Build history of the part. All positions in model axes, mm. Face numbers are marked on the shaded views. A direction names the side the tool comes from. Round coordinates to 2 decimals unless told otherwise and drop trailing zeros. Write each loop counter-clockwise with the first axis right and the second up, starting at its lowest first coordinate (ties: lowest second). Pieces come first, ordered by that corner, then holes.
1) Saw through at C-C (x = -38.5). Write the cut outline in (y, z).
2) Saw through at A-A (x = -62.5). Write the cut outline in (y, z), plus the area to 3 significant figures.
3) Which spindle directions (+Z, -Z, +X, -X, +Y, -Y) get a long thin tool onto all of the face, cutting with end or side? Do the marked faces 5 and 6. Say none if no direction does.
4) Pull direction X, two halves, no side cores. Call the marked faces 1, 2, 3 and 4: +X half, -X half, draft (parallel to the pull), parting line (faces both ways), or undercut.
5) Flat gauge pins, fed straight in: pin 1 (1.5 mm diameter, centred on x = 10.5, z = 7, fed in from -Y); pin 2 (2.5 mm diameter, centred on x = 56, z = 4, fed in from +Y); pin 3 (3 mm diameter, centred on x = 8.5, z = 4, fed in from -Y). Where does each tip first touch, or does it go through?
6) Wall check: probe 1 along X at (y, z) = (3.25, 2); probe 2 along Y at (x, z) = (-55.5, 2.25); probe 3 along Y at (x, z) = (-51, 2.5). Give the ranges that are in metal, low to high.
7) Saw through at B-B (y = 7). Write the cut outline in (x, z), plus the area to 3 significant figures.
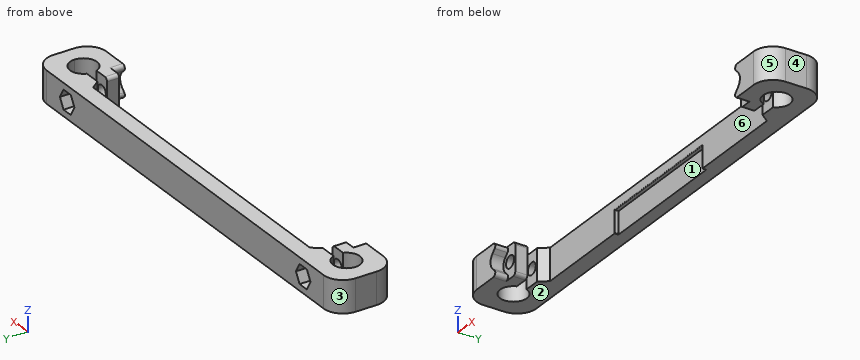
from build123d import *

# Parameters (mm, degrees)
SALIENTE_EXTRUIR1_DEPTH = 10
CROQUIS2_R              = 1.9
CORTAR_EXTRUIR1_DEPTH   = 25
CORTAR_EXTRUIR5_DEPTH   = 74.087139772
CROQUIS8_W              = 5.376990951
CROQUIS8_H              = 7.8
CORTAR_EXTRUIR6_DEPTH   = 74.087139772
CORTAR_EXTRUIR7_DEPTH   = 4.25
CROQUIS10_R             = 1.9
CORTAR_EXTRUIR8_DEPTH   = 4
REDONDEO1_R             = 1
CROQUIS11_W             = 41.47
CROQUIS11_H             = 14
CORTAR_EXTRUIR9_DEPTH   = 1.2
REDONDEO2_R             = 0.2


with BuildPart() as part:
    # Croquis1 → Saliente-Extruir1 (new body)
    with BuildSketch(Plane.XY):
        with BuildLine():
            Line((65.8, 9.3), (-65.8, 9.3))
            ThreePointArc((-65.8, 9.3), (-70.042640687, 7.542640687), (-71.8, 3.3))
            Line((-71.8, 3.3), (-71.8, -3.3))
            ThreePointArc((-71.8, -3.3), (-70.042640687, -7.542640687), (-65.8, -9.3))
            Line((-65.8, -9.3), (-48.2, -9.3))
            Line((-48.2, -9.3), (-48.2, -1.5))
            Line((-48.2, -1.5), (-58.576990951, -1.5))
            ThreePointArc((-58.576990951, -1.5), (-66.7, 0), (-58.576990951, 1.5))
            Line((-58.576990951, 1.5), (-46.2, 1.5))
            Line((-46.2, 1.5), (-46.2, -9.3))
            Line((-46.2, -9.3), (46.2, -9.3))
            Line((46.2, -9.3), (46.2, 1.5))
            Line((46.2, 1.5), (58.576990951, 1.5))
            ThreePointArc((58.576990951, 1.5), (63.26268014, 4.130171789), (66.7, 0))
            ThreePointArc((66.7, 0), (63.26268014, -4.130171789), (58.576990951, -1.5))
            Line((58.576990951, -1.5), (48.2, -1.5))
            Line((48.2, -1.5), (48.2, -9.3))
            Line((48.2, -9.3), (65.8, -9.3))
            ThreePointArc((65.8, -9.3), (70.042640687, -7.542640687), (71.8, -3.3))
            Line((71.8, -3.3), (71.8, 3.3))
            ThreePointArc((71.8, 3.3), (70.042640687, 7.542640687), (65.8, 9.3))
        make_face()
    extrude(amount=SALIENTE_EXTRUIR1_DEPTH)

    # Croquis2 → Cortar-Extruir1 (cut, symmetric)
    with BuildSketch(Plane.XZ.offset(-1.5)):
        with Locations(Location((-56.076990951, 5, 0), (0, 0, 180))):
            Circle(CROQUIS2_R)
        with Locations(Location((56.076990951, 5, 0), (0, 0, 180))):
            Circle(CROQUIS2_R)
    extrude(amount=CORTAR_EXTRUIR1_DEPTH, both=True, mode=Mode.SUBTRACT)

    # Croquis7 → Cortar-Extruir5 (cut, through all)
    with BuildSketch(Plane(origin=(0, 0, 0), x_dir=(-1, 0, 0), z_dir=(0, 0, -1))):
        Polygon((51.5, 4.2), (53.576990951, 1.5), (46.2, 1.5), (46.2, -9.3), (-46.2, -9.3), (-46.2, 1.5), (-53.576990951, 1.5), (-51.5, 4.2), align=None)
    extrude(amount=-CORTAR_EXTRUIR5_DEPTH, mode=Mode.SUBTRACT)

    # Croquis8 → Cortar-Extruir6 (cut, through all)
    with BuildSketch(Plane(origin=(0, 0, 0), x_dir=(-1, 0, 0), z_dir=(0, 0, -1))):
        with Locations((50.888495476, -5.4)):
            Rectangle(CROQUIS8_W, CROQUIS8_H)
        with Locations((-50.888495476, -5.4)):
            Rectangle(CROQUIS8_W, CROQUIS8_H)
    extrude(amount=-CORTAR_EXTRUIR6_DEPTH, mode=Mode.SUBTRACT)

    # Croquis5 → Cortar-Extruir7 (cut)
    with BuildSketch(Plane(origin=(0, 9.3, 0), x_dir=(1, 0, 0), z_dir=(0, 1, 0))):
        Polygon((-52.612889336, -5), (-54.344940143, -2), (-57.809041758, -2), (-59.541092566, -5), (-57.809041758, -8), (-54.344940143, -8), align=None)
        Polygon((59.541092566, -5), (57.809041758, -2), (54.344940143, -2), (52.612889336, -5), (54.344940143, -8), (57.809041758, -8), align=None)
    extrude(amount=-CORTAR_EXTRUIR7_DEPTH, mode=Mode.SUBTRACT)

    # Croquis10 → Cortar-Extruir8 (cut)
    # profile 1 of 2: a face of its own
    with BuildSketch(Plane.XZ.offset(9.3)):
        with BuildLine():
            Line((-53.576990951, 10), (-55.566305742, 10))
            Line((-55.566305742, 10), (-58.321648346, 7.244657395))
            ThreePointArc((-58.321648346, 7.244657395), (-59.251415882, 5), (-58.321648346, 2.755342605))
            Line((-58.321648346, 2.755342605), (-55.566305742, 0))
            Line((-55.566305742, 0), (-53.576990951, 0))
            Line((-53.576990951, 0), (-53.576990951, 10))
        make_face()
        with Locations((-56.076990951, 5)):
            Circle(CROQUIS10_R, mode=Mode.SUBTRACT)
    # profile 2 of 2: a face of its own
    with BuildSketch(Plane.XZ.offset(9.3)):
        with BuildLine():
            Line((58.321648346, 7.244657395), (55.566305742, 10))
            Line((55.566305742, 10), (53.576990951, 10))
            Line((53.576990951, 10), (53.576990951, 0))
            Line((53.576990951, 0), (55.566305742, 0))
            Line((55.566305742, 0), (58.321648346, 2.755342605))
            ThreePointArc((58.321648346, 2.755342605), (59.251415882, 5), (58.321648346, 7.244657395))
        make_face()
        with Locations((56.076990951, 5)):
            Circle(CROQUIS10_R, mode=Mode.SUBTRACT)
    extrude(amount=-CORTAR_EXTRUIR8_DEPTH, mode=Mode.SUBTRACT)

    # Redondeo1
    redondeo1_edges = [part.edges().sort_by_distance(p)[0] for p in [
        (53.576990951, -3.4, 10),
        (53.576990951, -3.4, 0),
        (-53.576990951, -3.4, 0),
        (-53.576990951, -3.4, 10),
        (-55.566305742, -7.3, 0),
        (-55.566305742, -7.3, 10),
        (55.566305742, -7.3, 0),
        (55.566305742, -7.3, 10),
    ]]
    fillet(redondeo1_edges, radius=REDONDEO1_R)

    # Croquis11 → Cortar-Extruir9 (cut)
    with BuildSketch(Plane.XZ.offset(-4.2)):
        Rectangle(CROQUIS11_W, CROQUIS11_H)
    extrude(amount=-CORTAR_EXTRUIR9_DEPTH, mode=Mode.SUBTRACT)

    # Redondeo2
    redondeo2_edges = [part.edges().sort_by_distance(p)[0] for p in [
        (20.735, 4.2, 3.5),
        (-20.735, 4.2, 3.5),
        (0, 4.2, 7),
        (-20.735, 4.8, 0),
        (20.735, 4.8, 0),
    ]]
    fillet(redondeo2_edges, radius=REDONDEO2_R)


solid = part.part
Evaluation:
1. outline: (4.2, 0) - (9.3, 0) - (9.3, 10) - (4.2, 10) - close
2. outline: (-9.3, 0) - (-4.2, 0) - (-4.2, 10) - (-9.3, 10) - close; (4.2, 0) - (9.3, 0) - (9.3, 10) - (4.2, 10) - close
2. area: 102 mm2
3. face 5: +Z, -Z, +X, -Y
3. face 6: +Z, -Z, -Y
4. face 1: undercut
4. face 2: draft
4. face 3: -X half
4. face 4: +X half
5. pin 1: stops at y = 4.2
5. pin 2: stops at y = 5.05
5. pin 3: stops at y = 5.4
6. probe 1: x = -71.8 to -65.16, -59.84 to -52.23, 52.23 to 59.84, 65.16 to 71.8
6. probe 2: y = -5.3 to -1.5, 1.5 to 5.05
6. probe 3: y = 4.2 to 9.3
7. outline: (-70.52, 0) - (70.52, 0) - (70.52, 10) - (-70.52, 10) - close; hole (-59.54, 5) - (-57.81, 2) - (-54.34, 2) - (-52.61, 5) - (-54.34, 8) - (-57.81, 8) - close; hole (52.61, 5) - (54.34, 2) - (57.81, 2) - (59.54, 5) - (57.81, 8) - (54.34, 8) - close
7. area: 1,350 mm2
